Verification items for the finished model (mm, model axes). Give positions to 0.01 mm unless a question says otherwise; leave off trailing zeros. Use CSV: the item, a comma, the result in double quotes.
from build123d import *

# Parameters (mm, degrees)
SKETCH_1_W      = 550
SKETCH_1_H      = 56
SKETCH_1_R      = 3.05
SKETCH_1_R_2    = 1.6
SKETCH_1_R_3    = 1.741142055
SKETCH_1_R_4    = 1.469666532
SKETCH_1_R_5    = 1.619836661
SKETCH_1_R_6    = 1.494419625
SKETCH_1_R_7    = 1.78071741
EXTRUDE_1_DEPTH = 5
FILLET_1_R      = 10


with BuildPart() as part:
    # 草图1 → 凸台-拉伸1 (new body)
    with BuildSketch(Plane(origin=(0, 0, 0), x_dir=(1, 0, 0), z_dir=(0, 1, 0))):
        with Locations((0, 28)):
            Rectangle(SKETCH_1_W, SKETCH_1_H)
        with Locations(Location((-265.5, 43, 0), (0, 0, 270))):
            Circle(SKETCH_1_R, mode=Mode.SUBTRACT)
        with Locations(Location((-265.5, 13, 0), (0, 0, 270))):
            Circle(SKETCH_1_R, mode=Mode.SUBTRACT)
        with Locations(Location((265.5, 13, 0), (0, 0, 90))):
            Circle(SKETCH_1_R, mode=Mode.SUBTRACT)
        with Locations(Location((265.5, 43, 0), (0, 0, 90))):
            Circle(SKETCH_1_R, mode=Mode.SUBTRACT)
        with Locations(Location((239.176550925, 48, 0), (0, 0, 270))):
            Circle(SKETCH_1_R_2, mode=Mode.SUBTRACT)
        with Locations(Location((239.176550925, 8, 0), (0, 0, 270))):
            Circle(SKETCH_1_R_2, mode=Mode.SUBTRACT)
        with Locations(Location((121.376550925, 48, 0), (0, 0, 270))):
            Circle(SKETCH_1_R_2, mode=Mode.SUBTRACT)
        with Locations(Location((121.376550925, 8, 0), (0, 0, 270))):
            Circle(SKETCH_1_R_2, mode=Mode.SUBTRACT)
        with Locations(Location((-170.393257171, 51.376890861, 0), (0, 0, 270))):
            Circle(SKETCH_1_R_2, mode=Mode.SUBTRACT)
        with Locations(Location((-219.393257171, 51.376890861, 0), (0, 0, 270))):
            Circle(SKETCH_1_R_2, mode=Mode.SUBTRACT)
        with Locations(Location((-224.393257171, 51.376890861, 0), (0, 0, 270))):
            Circle(SKETCH_1_R_2, mode=Mode.SUBTRACT)
        with Locations(Location((-224.393257171, 3.414613144, 0), (0, 0, 270))):
            Circle(SKETCH_1_R_3, mode=Mode.SUBTRACT)
        with Locations(Location((-165.393257171, 51.376890861, 0), (0, 0, 270))):
            Circle(SKETCH_1_R_2, mode=Mode.SUBTRACT)
        with Locations(Location((-165.393257171, 3.414613144, 0), (0, 0, 270))):
            Circle(SKETCH_1_R_3, mode=Mode.SUBTRACT)
        with Locations(Location((-132.483237063, 53, 0), (0, 0, 270))):
            Circle(SKETCH_1_R_4, mode=Mode.SUBTRACT)
        with Locations(Location((-132.483237063, 3, 0), (0, 0, 270))):
            Circle(SKETCH_1_R_5, mode=Mode.SUBTRACT)
        with Locations(Location((-36.483237063, 53, 0), (0, 0, 270))):
            Circle(SKETCH_1_R_6, mode=Mode.SUBTRACT)
        with Locations(Location((-36.483237063, 3, 0), (0, 0, 270))):
            Circle(SKETCH_1_R_7, mode=Mode.SUBTRACT)
        with BuildLine():
            Line((-147.397504582, 49.857044682), (-147.397504582, 40.853271456))
            ThreePointArc((-147.397504582, 40.853271456), (-149.731816159, 38.518959879), (-152.066127736, 40.853271456))
            Line((-152.066127736, 40.853271456), (-152.066127736, 49.857044682))
            ThreePointArc((-152.066127736, 49.857044682), (-149.731816159, 52.191356259), (-147.397504582, 49.857044682))
        make_face(mode=Mode.SUBTRACT)
        with BuildLine():
            Line((-147.730977664, 15.67605373), (-147.730977664, 8))
            ThreePointArc((-147.730977664, 8), (-149.731816159, 5.999161505), (-151.732654654, 8))
            Line((-151.732654654, 8), (-151.732654654, 15.67605373))
            ThreePointArc((-151.732654654, 15.67605373), (-149.731816159, 17.676892225), (-147.730977664, 15.67605373))
        make_face(mode=Mode.SUBTRACT)
        with BuildLine():
            Line((-233.443564049, 49.857044682), (-233.443564049, 39.145889274))
            ThreePointArc((-233.443564049, 39.145889274), (-235.604469624, 36.984983699), (-237.765375198, 39.145889274))
            Line((-237.765375198, 39.145889274), (-237.765375198, 49.857044682))
            ThreePointArc((-237.765375198, 49.857044682), (-235.604469624, 52.017950257), (-233.443564049, 49.857044682))
        make_face(mode=Mode.SUBTRACT)
        with BuildLine():
            Line((-232.723262191, 21.138342821), (-232.723262191, 9.613513091))
            ThreePointArc((-232.723262191, 9.613513091), (-235.604469624, 6.732305658), (-238.485677056, 9.613513091))
            Line((-238.485677056, 9.613513091), (-238.485677056, 21.138342821))
            ThreePointArc((-238.485677056, 21.138342821), (-235.604469624, 24.019550253), (-232.723262191, 21.138342821))
        make_face(mode=Mode.SUBTRACT)
        with BuildLine():
            Line((15.525688633, 46), (5.525688633, 46))
            ThreePointArc((5.525688633, 46), (3.525688633, 48), (5.525688633, 50))
            Line((5.525688633, 50), (15.525688633, 50))
            ThreePointArc((15.525688633, 50), (17.525688633, 48), (15.525688633, 46))
        make_face(mode=Mode.SUBTRACT)
        with BuildLine():
            Line((84.556283314, 46), (74.556283314, 46))
            ThreePointArc((74.556283314, 46), (72.556283314, 48), (74.556283314, 50))
            Line((74.556283314, 50), (84.556283314, 50))
            ThreePointArc((84.556283314, 50), (86.556283314, 48), (84.556283314, 46))
        make_face(mode=Mode.SUBTRACT)
        with BuildLine():
            Line((15.525688633, 6), (5.525688633, 6))
            ThreePointArc((5.525688633, 6), (3.525688633, 8), (5.525688633, 10))
            Line((5.525688633, 10), (15.525688633, 10))
            ThreePointArc((15.525688633, 10), (17.525688633, 8), (15.525688633, 6))
        make_face(mode=Mode.SUBTRACT)
        with BuildLine():
            Line((84.556283314, 6), (74.556283314, 6))
            ThreePointArc((74.556283314, 6), (72.556283314, 8), (74.556283314, 10))
            Line((74.556283314, 10), (84.556283314, 10))
            ThreePointArc((84.556283314, 10), (86.556283314, 8), (84.556283314, 6))
        make_face(mode=Mode.SUBTRACT)
        with BuildLine():
            Line((169.833189375, 52), (187.927295943, 52))
            ThreePointArc((187.927295943, 52), (189.927295943, 50), (187.927295943, 48))
            Line((187.927295943, 48), (169.833189375, 48))
            ThreePointArc((169.833189375, 48), (167.833189375, 50), (169.833189375, 52))
        make_face(mode=Mode.SUBTRACT)
        with BuildLine():
            Line((169.833189375, 8), (187.927295943, 8))
            ThreePointArc((187.927295943, 8), (189.927295943, 6), (187.927295943, 4))
            Line((187.927295943, 4), (169.833189375, 4))
            ThreePointArc((169.833189375, 4), (167.833189375, 6), (169.833189375, 8))
        make_face(mode=Mode.SUBTRACT)
    extrude(amount=EXTRUDE_1_DEPTH)

    # 圆角1
    fillet_1_edges = [part.edges().sort_by_distance(p)[0] for p in [
        (-275, 2.5, -56),
        (275, 2.5, -56),
        (275, 2.5, 0),
        (-275, 2.5, 0),
    ]]
    fillet(fillet_1_edges, radius=FILLET_1_R)


solid = part.part
(1) Scan lines: L1, parallel to X at y = 1.15, z = -13; L2, parallel to Z at x = 175.5, y = 2.55; L3, parallel to Z at x = 73, y = 2.35. Record each from-to range of solid material in increasing order. Write a range as from..to.
Calculated:
L1,"x = -275..-268.55, -262.45..-238.49, -232.72..-151.73, -147.73..262.45, 268.55..275"
L2,"z = -56..-52, -48..-8, -4..0"
L3,"z = -56..-49.26, -46.74..-9.26, -6.74..0"
(2) Depth check by flat-ended pin: pin 1 Ø3 at (x, z) = (-219.39, -51.38) entering from -Y. Enter the tip coordinate at first touch or a pass-through.
Calculated:
pin 1,"passes through"
(3) Section check A-A on y = 2.1. Count the separate pieces of the cut face and the enclosed holes in it, plus the area to 3 significant figures.
Calculated:
separate pieces,"1"
enclosed holes,"28"
area,"29,800 mm²"
